```python
from build123d import *

# Parameters (mm, degrees)
SKETCH1_W               = 60
SKETCH1_H               = 35
BOSS_EXTRUDE1_DEPTH     = 10
SKETCH2_W               = 22
SKETCH2_H               = 10
CUT_EXTRUDE1_DEPTH      = 19
SKETCH3_W               = 22
SKETCH3_H               = 10
CUT_EXTRUDE2_DEPTH      = 29
SKETCH5_R               = 1.6
CUT_EXTRUDE4_DEPTH      = 71.178344238
FILLET1_R               = 3
FILLET2_R               = 3
SKETCH7_W               = 12
SKETCH7_H               = 10
BOSS_EXTRUDE2_DEPTH     = 3
CUT_EXTRUDE5_DEPTH      = 3
CUT_EXTRUDE5_DEPTH_BACK = 15
SKETCH6_R               = 1.5
FILLET3_R               = 4


with BuildPart() as part:
    # Sketch1 → Boss-Extrude1 (new body)
    with BuildSketch(Plane(origin=(0, 0, 0), x_dir=(1, 0, 0), z_dir=(0, 1, 0))):
        with Locations((30, -17.5)):
            Rectangle(SKETCH1_W, SKETCH1_H)
    extrude(amount=BOSS_EXTRUDE1_DEPTH)

    # Sketch2 → Cut-Extrude1 (cut)
    with BuildSketch(Plane(origin=(60, 0, 0), x_dir=(0, 0, -1), z_dir=(1, 0, 0))):
        with Locations((-17.5, 5)):
            Rectangle(SKETCH2_W, SKETCH2_H)
    extrude(amount=-CUT_EXTRUDE1_DEPTH, mode=Mode.SUBTRACT)

    # Sketch3 → Cut-Extrude2 (cut)
    with BuildSketch(Plane.ZY):
        with Locations((17.5, 5)):
            Rectangle(SKETCH3_W, SKETCH3_H)
    extrude(amount=-CUT_EXTRUDE2_DEPTH, mode=Mode.SUBTRACT)

    # Sketch5 → Cut-Extrude4 (cut, through all)
    with BuildSketch(Plane.XY.offset(35)):
        with Locations((5, 5)):
            Circle(SKETCH5_R)
        with Locations((55, 5)):
            Circle(SKETCH5_R)
    extrude(amount=-CUT_EXTRUDE4_DEPTH, mode=Mode.SUBTRACT)

    # Fillet1
    fillet1_edges = [part.edges().sort_by_distance(p)[0] for p in [
        (60, 10, 31.75),
        (60, 0, 3.25),
        (60, 10, 3.25),
        (0, 0, 31.75),
        (0, 10, 31.75),
        (0, 10, 3.25),
        (60, 0, 31.75),
        (0, 0, 3.25),
    ]]
    fillet(fillet1_edges, radius=FILLET1_R)

    # Fillet2
    fillet2_edges = [part.edges().sort_by_distance(p)[0] for p in [
        (41, 5, 28.5),
        (41, 5, 6.5),
        (29, 5, 6.5),
        (29, 5, 28.5),
    ]]
    fillet(fillet2_edges, radius=FILLET2_R)

    # Sketch7 → Boss-Extrude2 (add)
    with BuildSketch(Plane.XY.offset(35)):
        with Locations((35, 5)):
            Rectangle(SKETCH7_W, SKETCH7_H)
    extrude(amount=BOSS_EXTRUDE2_DEPTH)

    # Sketch6 → Cut-Extrude5 (cut, two sides: drawn at the far end of the back side and taken through both)
    with BuildSketch(Plane.XY.offset(35).offset(-CUT_EXTRUDE5_DEPTH_BACK)):
        with Locations((34.5, 5)):
            Circle(SKETCH6_R)
    extrude(amount=CUT_EXTRUDE5_DEPTH + CUT_EXTRUDE5_DEPTH_BACK, mode=Mode.SUBTRACT)

    # Fillet3
    # the kernel refuses this fillet: 4 mm, written as the material it adds along each edge
    with BuildSketch(Plane(origin=(41, 10, 35), x_dir=(0, 0, 1), z_dir=(0, -1, 0))) as fillet3_piece_1:
        with BuildLine():
            CenterArc((4, -3.872983346), FILLET3_R, 104.477512186, 75.522487814)
            Line((0, -3.872983346), (-0.08, -3.872983346))
            Line((-0.08, -3.872983346), (-0.08, 0))
            Line((-0.08, 0), (0, 0.08))
            ThreePointArc((0, 0.08), (1.5, 0.08), (2.98, 0.077459667))
            Line((2.98, 0.077459667), (3, 0))
        make_face()
    extrude(amount=10)
    with BuildSketch(Plane(origin=(29, 0, 35), x_dir=(-1, 0, 0), z_dir=(0, 1, 0))) as fillet3_piece_2:
        with BuildLine():
            CenterArc((3.872983346, 4), FILLET3_R, 194.477512186, 75.522487814)
            Line((0, 3), (-0.077459667, 2.98))
            ThreePointArc((-0.077459667, 2.98), (-0.08, 1.5), (-0.08, 0))
            Line((-0.08, 0), (0, -0.08))
            Line((0, -0.08), (3.872983346, -0.08))
            Line((3.872983346, -0.08), (3.872983346, 0))
        make_face()
    extrude(amount=10)


solid = part.part
```
Input: part model. Units: mm. Frame: model coordinates. A direction names the side the tool comes from. Give positions to 0.01 mm unless a question says otherwise; leave off trailing zeros. Order: outer loops, then holes, each group sorted by start corner. A loop starts at its lowest first (then second) coordinate and runs counter-clockwise, first axis right, second up. Notation, with made-up numbers: (88, 49) -> (111, 49) arc R8 ccw to (111, 61) -> close; hole circle Ø1 at (-25.5, 48). An arc over 180 degrees is marked (long way). Write each question's results on one line, items separated by ' | '. Start each with the question number.
Item 1: Cut plane A-A on x = 50. Return the cut outline in (y, z).
Item 2: Contact query for flat-ended pins moving along their axis: P1, Ø1.5, axis at y = 8.5, z = 25, coming from the -X side; P2, Ø6, axis at y = 7, z = 20, coming from the +X side; P3, Ø5, axis at y = 8.5, z = 10, coming from the -X side. Output: stop coordinate, or through.
Item 3: Line query: line 1 (Z direction, x = 50.5, y = 2.25); line 2 (Y direction, x = 55, z = 4.5); line 3 (Y direction, x = 34.5, z = 25.25). Output: solid intervals per line, ascending.
Item 4: Cut plane C-C on x = 6. Return the cut outline in (y, z), then the cut area to 3 significant figures.
Item 5: Cut plane B-B on z = 31. Return the cut outline in (x, y), then the cut area to 3 significant figures.
Item 6: Mould query, pull axis Y, two halves, no side actions, for faces 4 (the flat face through (52, 5, 28.5)), 5 (the cylindrical face through (33.3, 4.1, 28.9)), 6 (the cylindrical face through (0.9, 9.14, 3.2)), 7 (the cylindrical face through (56.48, 4.39, 31.8)). Classes: pulls with the +Y half, pulls with the -Y half, needs draft (parallel to the pull), parting line crosses it, or undercut.
Item 7: Cut plane D-D on y = 1.5. Return the cut outline in (x, z).
Item 8: Set-up query: faces 1 (the flat face through (41, 5, 18)), 2 (the flat face through (12, 5, 35)), 3 (the flat face through (29, 5, 17)). Return all of +Z, -Z, +X, -X, +Y, -Y with unobstructed straight access to the full face (end or side cutting, diameter ignored); none if empty.
Established:
1) outline: (0, 0) -> (10, 0) -> (10, 6.5) -> (0, 6.5) -> close; (0, 28.5) -> (10, 28.5) -> (10, 35) -> (0, 35) -> close
2) P1: x = 28.99 | P2: x = 41 | P3: x = 28.24
3) line 1: 0 to 6.5, 28.5 to 35 | line 2: 0 to 3.4, 6.6 to 10 | line 3: 0 to 3.5, 6.5 to 10
4) outline: (0, 0) -> (3.75, 0) -> (3.75, 6.5) -> (0, 6.5) -> close; (0, 28.5) -> (3.75, 28.5) -> (3.75, 35) -> (0, 35) -> close; (6.25, 0) -> (10, 0) -> (10, 6.5) -> (6.25, 6.5) -> close; (6.25, 28.5) -> (10, 28.5) -> (10, 35) -> (6.25, 35) -> close | area: 97.5 mm^2
5) outline: (0, 3) arc R3 ccw to (3, 0) -> (57, 0) arc R3 ccw to (60, 3) -> (60, 7) arc R3 ccw to (57, 10) -> (3, 10) arc R3 ccw to (0, 7) -> close; hole circle Ø3.2 at (5, 5); hole circle Ø3 at (34.5, 5); hole circle Ø3.2 at (55, 5) | area: 569 mm^2
6) face 4: needs draft | face 5: undercut | face 6: pulls with the +Y half | face 7: undercut
7) outline: (0.4, 0) -> (59.6, 0) -> (59.6, 6.5) -> (44, 6.5) arc R3 cw to (41, 9.5) -> (41, 25.5) arc R3 cw to (44, 28.5) -> (59.6, 28.5) -> (59.6, 35) -> (44.87, 35) arc R4 cw to (41, 38) -> (29, 38) arc R4 cw to (25.13, 35) -> (0.4, 35) -> (0.4, 28.5) -> (26, 28.5) arc R3 cw to (29, 25.5) -> (29, 9.5) arc R3 cw to (26, 6.5) -> (0.4, 6.5) -> close
8) face 1: +X, +Y, -Y | face 2: +Z, -X, +Y, -Y | face 3: -X, +Y, -Y
